Part model, mm, in its own coordinate system. Face numbers are marked on the shaded views. A direction names the side the tool comes from. Give positions to 0.01 mm unless a question says otherwise; leave off trailing zeros. Order: outer loops, then holes, each group sorted by start corner. A loop starts at its lowest first (then second) coordinate and runs counter-clockwise, first axis right, second up. Notation, with made-up numbers: (-26.5, 75) - (16.5, 75) arc R29 ccw to (16.5, 110) - close; hole circle Ø3 at (-22, -14.5). An arc over 180 degrees is marked (long way). Use one line per item in the form item = value. Start each with the question number.
1. Drill centre lines: line 1 (Z direction, x = 18, y = 164.5); line 2 (Z direction, x = 0, y = 11.5); line 3 (X direction, y = 12, z = 0). Where is each one in solid material? Low to high.
2. Band-saw the part on A-A, the plane x = 0. List the corners of the cut face in (y, z), plus the area to 3 significant figures.
3. Tool access for the marked faces 4, 5, 6 and 7: list every direction of +Z, -Z, +X, -X, +Y, -Y with a clear straight run to the whole face (end or side of a thin tool).
4. Pull direction Z, two halves, no side cores. Call the marked faces 1, 2 and 3: +Z half, -Z half, draft (parallel to the pull), parting line (faces both ways), or undercut.
5. Pin check, flat tips, straight feed: P1, Ø8, axis at x = 6.5, z = -4, coming from the +Y side; P2, Ø3, axis at x = -17, y = 93, coming from the +Z side; P3, Ø12, axis at x = 3, z = -1, coming from the -Y side; P4, Ø3, axis at x = 11, z = -19.5, coming from the -Y side. Stop position of each tip, or through.
6. Band-saw the part on D-D, the plane x = 8. List the corners of the cut face in (y, z), plus the area to 3 significant figures.
7. Band-saw the part on B-B, the plane z = -12. List the corners of the cut face in (x, y).
8. Band-saw the part on C-C, the plane y = 40. List the corners of the cut face in (x, z), plus the area to 3 significant figures.
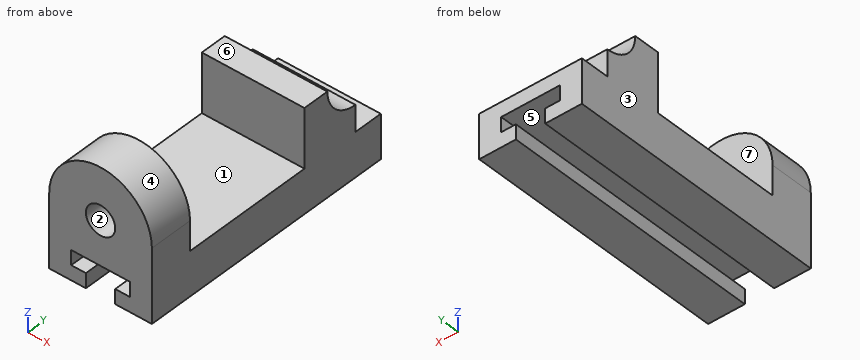
Autodesk Fusion 360 part; units mm, degrees
sketch "Sketch1" plane through (0, 0, 0) normal (0, 1, 0) x (1, 0, 0)
  circle A0 centre (0, 0) radius 10
  line L0 (-35, 0) -> (-35, 50)
  line L1 (35, 50) -> (35, 0)
  arc A1 (-35, 0) -> (35, 0) centre (0, 0) ccw
  line L2 (-10, 50) -> (-10, 40)
  line L3 (-20, 40) -> (-10, 40)
  line L4 (-20, 40) -> (-20, 30)
  line L5 (20, 30) -> (20, 40)
  line L6 (20, 40) -> (10, 40)
  line L7 (10, 40) -> (10, 50)
  line L8 (-20, 30) -> (-18.0278, 30)
  line L9 (18.0278, 30) -> (20, 30)
  line L10 (-18.0278, 30) -> (18.0278, 30)
  line L11 (-35, 50) -> (-10, 50)
  line L12 (10, 50) -> (35, 50)
  dimension "d1" = 70
  dimension "d2" = 50
  dimension "d3" = 70
  dimension "d4" = 90
  dimension "d5" = 90
extrude "Extrude1" add sketch "Sketch1" along normal blind 30
sketch "Sketch2" plane through (0, 30, 0) normal (0, 1, 0) x (-1, 0, 0)
  circle A0 centre (0, 0) radius 10
  line L0 (20, -40) -> (10, -40)
  line L1 (10, -40) -> (10, -50)
  line L2 (10, -50) -> (35, -50)
  line L3 (35, -50) -> (35, 0)
  arc A1 (35, 0) -> (-35, 0) centre (0, 0) ccw
  line L4 (-35, 0) -> (-35, -50)
  line L5 (-35, -50) -> (-10, -50)
  line L6 (-10, -50) -> (-10, -40)
  line L7 (-10, -40) -> (-20, -40)
  line L8 (-20, -40) -> (-20, -30)
  line L9 (-20, -30) -> (20, -30)
  line L10 (20, -30) -> (20, -40)
  line L11 (-35, -50) -> (35, -50)
  line L12 (35, -50) -> (35, -20)
  line L13 (35, -20) -> (-35, -20)
  line L14 (-35, -20) -> (-35, -50)
extrude "Extrude2" add sketch "Sketch2" along normal blind 90 contours L0 L1 L2 L3 L4 L5 L6 L7 L8 L9 L10 L11 L12 L13 L14 | L0 L1 L6 L7 L8 L9 L10 L11
sketch "Sketch3" plane through (0, 120, 0) normal (0, 1, 0) x (-1, 0, 0)
  line L0 (-35, -20) -> (-35, -50)
  line L1 (-35, -50) -> (35, -50)
  line L2 (35, -50) -> (35, -20)
  line L3 (35, -20) -> (-35, -20)
  line L4 (-35, -50) -> (35, -50)
  line L5 (35, -50) -> (35, 20)
  line L6 (35, 20) -> (-35, 20)
  line L7 (-35, 20) -> (-35, -50)
  dimension "d10" = 70
  dimension "d11" = 70
extrude "Extrude3" add sketch "Sketch3" along normal blind 18
sketch "Sketch4" plane through (-35, 0, 0) normal (-1, 0, 0) x (0, -1, 0)
  line L0 (0, -50) -> (0, 0)
  line L1 (0, 0) -> (-30, 0)
  line L2 (-30, 0) -> (-30, -20)
  line L3 (-30, -20) -> (-120, -20)
  line L4 (-120, -20) -> (-120, 20)
  line L5 (-120, 20) -> (-138, 20)
  line L6 (-138, 20) -> (-138, -50)
  line L7 (-138, -50) -> (0, -50)
  line L8 (-138, -50) -> (-160, -50)
  line L9 (-160, -50) -> (-160, -2)
  line L10 (-138, 20) -> (-138, -50)
  arc A0 (-160, -2) -> (-138, 20) centre (-160, 20) ccw
  dimension "d14" = 22
extrude "Extrude4" add sketch "Sketch4" against normal blind 70 contours L6 L8 L9 L10 A0
sketch "Sketch5" plane through (0, 160, 0) normal (0, 1, 0) x (-1, 0, 0)
  line L0 (35, -50) -> (35, -2)
  line L1 (35, -2) -> (-35, -2)
  line L2 (-35, -2) -> (-35, -50)
  line L3 (-35, -50) -> (35, -50)
  line L4 (-35, -50) -> (35, -50)
  line L5 (35, -50) -> (35, -20)
  line L6 (35, -20) -> (-35, -20)
  line L7 (-35, -20) -> (-35, -50)
  dimension "d17" = 30
extrude "Extrude5" add sketch "Sketch5" along normal blind 20 contours L0 L2 L3 L4 L5 L6 L7
sketch "Sketch6" plane through (0, 0, 0) normal (0, -1, 0) x (1, 0, 0)
  circle A0 centre (0, 0) radius 10
  line L0 (-10, -40) -> (-20, -40)
  line L1 (-20, -40) -> (-20, -30)
  line L2 (-20, -30) -> (20, -30)
  line L3 (20, -30) -> (20, -40)
  line L4 (20, -40) -> (10, -40)
  line L5 (10, -40) -> (10, -50)
  line L6 (10, -50) -> (35, -50)
  line L7 (35, -50) -> (35, 0)
  arc A1 (35, 0) -> (-35, 0) centre (0, 0) ccw
  line L8 (-35, 0) -> (-35, -50)
  line L9 (-35, -50) -> (-10, -50)
  line L10 (-10, -50) -> (-10, -40)
  line L11 (-10, -50) -> (-10, -40)
  line L12 (-10, -40) -> (-20, -40)
  line L13 (-20, -40) -> (-20, -30)
  line L14 (-20, -30) -> (20, -30)
  line L15 (20, -30) -> (20, -40)
  line L16 (20, -40) -> (10, -40)
  line L17 (10, -40) -> (10, -50)
  line L18 (-10, -50) -> (10, -50)
extrude "Extrude6" cut sketch "Sketch6" against normal blind 210 contours L0 L1 L2 L3 L4 L5 L10 L11 L12 L13 L14 L15 L16 L17 L18
From the geometry:
q1.line_1 = -50 to -40, -30 to -20
q1.line_2 = -30 to -10, 10 to 35
q1.line_3 = -35 to -10, 10 to 35
q2.outline = (0, -30) - (180, -30) - (180, -20) - (160, -20) - (160, -2) arc R22 cw to (138, 20) - (120, 20) - (120, -20) - (30, -20) - (30, -10) - (0, -10) - close; (0, 10) - (30, 10) - (30, 35) - (0, 35) - close
q2.area = 4,070 mm²
q3.face_4 = +Z, -Y
q3.face_5 = +Y, -Y
q3.face_6 = +Z, +X, -X, +Y
q3.face_7 = +Z, +X, -X
q4.face_1 = +Z half
q4.face_2 = undercut
q4.face_3 = draft
q5.P1 = 160
q5.P2 = -20
q5.P3 = 120
q5.P4 = 0
q6.outline = (0, -30) - (180, -30) - (180, -20) - (160, -20) - (160, -2) arc R22 cw to (138, 20) - (120, 20) - (120, -20) - (30, -20) - (30, -6) - (0, -6) - close; (0, 6) - (30, 6) - (30, 34.07) - (0, 34.07) - close
q6.area = 4,280 mm²
q7.outline = (-35, 0) - (35, 0) - (35, 30) - (-35, 30) - close; (-35, 120) - (35, 120) - (35, 160) - (-35, 160) - close
q8.outline = (-35, -50) - (-10, -50) - (-10, -40) - (-20, -40) - (-20, -30) - (20, -30) - (20, -40) - (10, -40) - (10, -50) - (35, -50) - (35, -20) - (-35, -20) - close
q8.area = 1,500 mm²
